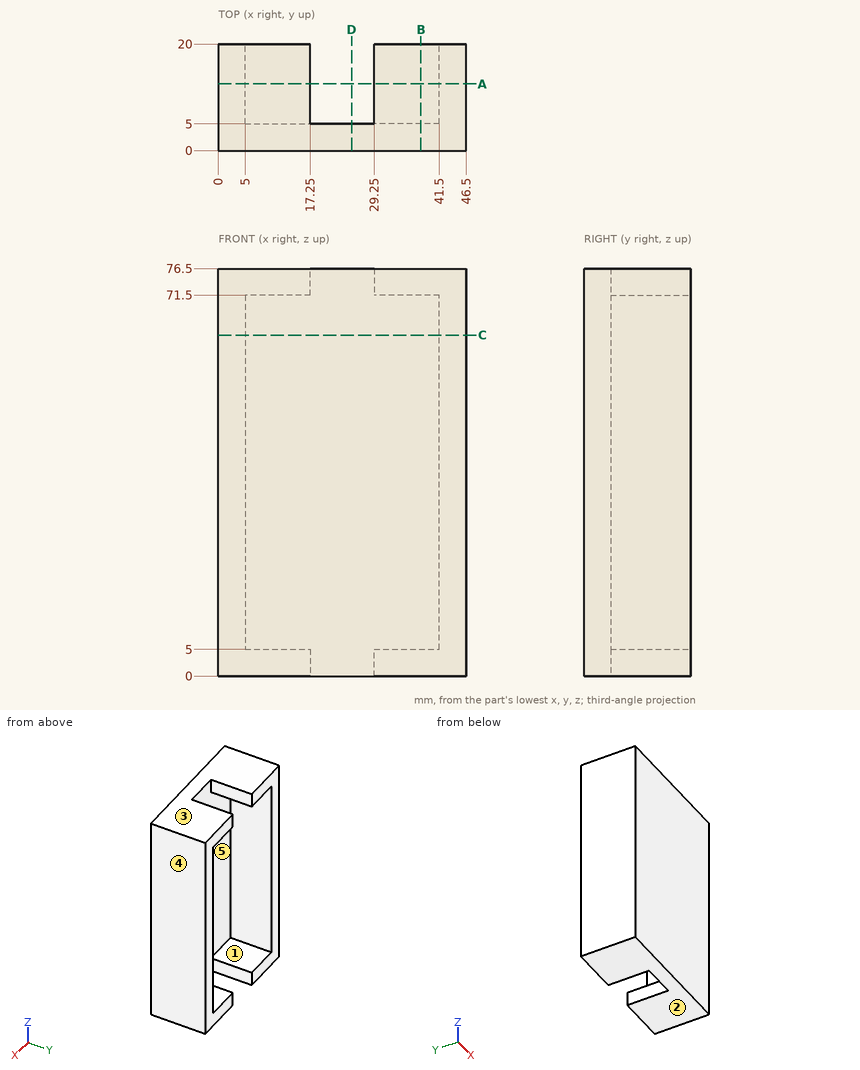
The drawing under review shows one solid part. Ordinate dimensions are in mm from its lowest x, y, z. A direction names the side the tool comes from. Coordinates: 2 decimals unless noted, no trailing zeros. Loops run counter-clockwise (first coordinate to the right, second up) from the corner with the lowest first, then second, coordinate; pieces in that order, holes last. Notation, with made-up numbers: (59.25, 59) -> (83.25, 59) arc R27 ccw to (83.25, 98) -> close; hole circle Ø9 at (1.25, 36). An arc over 180 degrees is marked (long way). Answer as a JSON object with one key per item and string values.
Q1. To check wall thickness, follow L1, parallel to Z at x = 6.5, y = 12.25; L2, parallel to X at y = 19, z = 25.5; L3, parallel to Y at x = 6, z = 39.5. State the ranges of each line that lie inside material, in increasing order.
Answer block:
{"L1": "z = 0 to 5, 71.5 to 76.5", "L2": "x = 0 to 5, 41.5 to 46.5", "L3": "y = 0 to 5"}
Q2. Clearance check with a flat-ended pin moving along its axis: pin 1 Ø5 at (x, z) = (14, 20.5) entering from +Y. State where the tip first meets the part, or that it passes through.
Answer block:
{"pin 1": "stops at y = 5"}
Q3. Take a section at D-D on x = 25. Give the boundary of the cut face in (y, z).
Answer block:
{"outline": "(0, 0) -> (5, 0) -> (5, 76.5) -> (0, 76.5) -> close"}
Q4. The part is to be moulded in two halves that separate along Z. For the marked faces 3, 4 and 5, say which applies: +Z half, -Z half, draft (parallel to the pull), parting line (faces both ways), or undercut.
Answer block:
{"face 3": "+Z half", "face 4": "draft", "face 5": "undercut"}
Q5. Take a section at C-C on z = 64. Give the boundary of the cut face in (x, y), plus the area to 4 significant figures.
Answer block:
{"outline": "(0, 0) -> (46.5, 0) -> (46.5, 20) -> (41.5, 20) -> (41.5, 5) -> (5, 5) -> (5, 20) -> (0, 20) -> close", "area": "382.5 mm^2"}
Q6. Tool access review of the marked faces 1 and 2: name each direction out of +Z, -Z, +X, -X, +Y, -Y from which nothing blocks a thin tool from reaching the whole face with its end or side.
Answer block:
{"face 1": "+Y", "face 2": "-Z, +X, -X, +Y, -Y"}
Q7. Take a section at A-A on y = 12.5. Give the boundary of the cut face in (x, z).
Answer block:
{"outline": "(0, 0) -> (17.25, 0) -> (17.25, 5) -> (5, 5) -> (5, 71.5) -> (17.25, 71.5) -> (17.25, 76.5) -> (0, 76.5) -> close; (29.25, 0) -> (46.5, 0) -> (46.5, 76.5) -> (29.25, 76.5) -> (29.25, 71.5) -> (41.5, 71.5) -> (41.5, 5) -> (29.25, 5) -> close"}
Q8. Take a section at B-B on x = 38. Give the boundary of the cut face in (y, z).
Answer block:
{"outline": "(0, 0) -> (20, 0) -> (20, 5) -> (5, 5) -> (5, 71.5) -> (20, 71.5) -> (20, 76.5) -> (0, 76.5) -> close"}
